Print and shaded views of the part. All mm, measured from the part's lowest x, y and z. Round coordinates to 2 decimals unless told otherwise and drop trailing zeros. Loops run counter-clockwise (first coordinate to the right, second up) from the corner with the lowest first, then second, coordinate; pieces in that order, holes last. Notation, with made-up numbers: (64.5, 35.25) -> (68.5, 35.25) arc R19 ccw to (68.5, 69.25) -> close; hole circle Ø4 at (17, 38.25). An arc over 180 degrees is marked (long way). Answer as CSV lines item,"result".
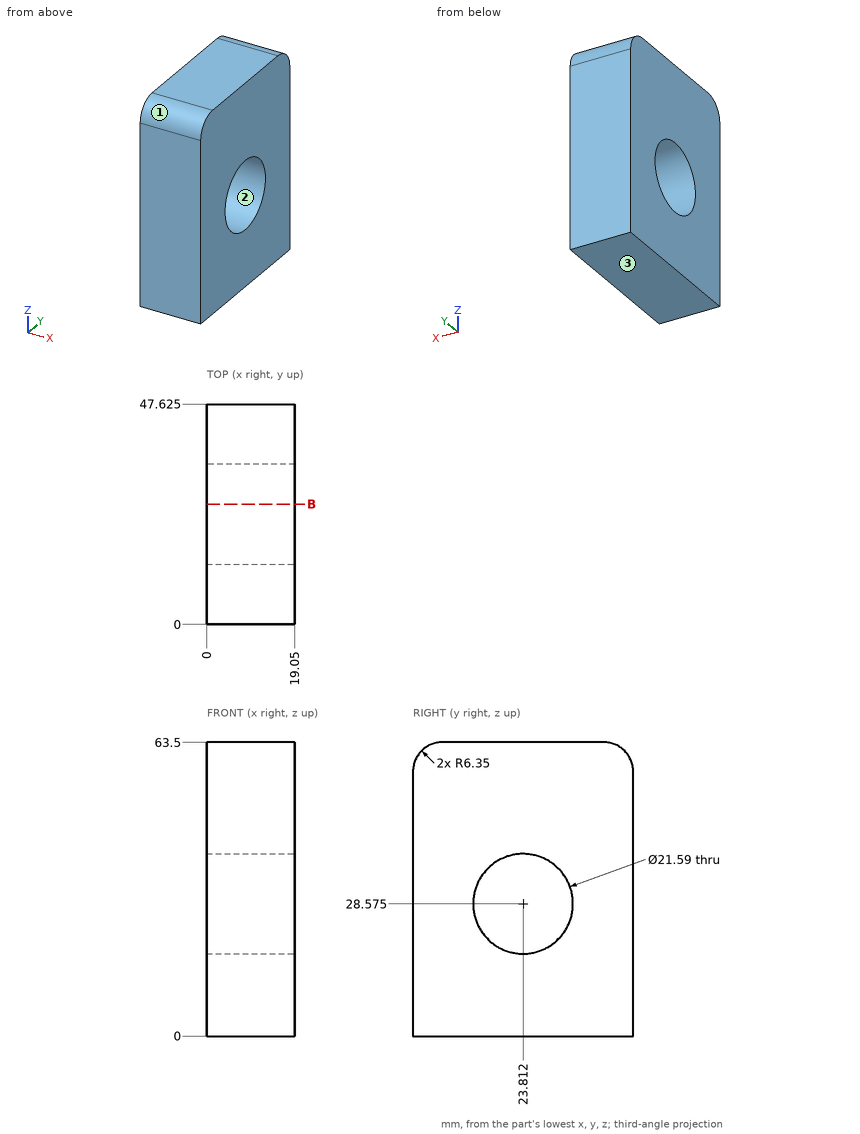
Q1. Drill centre lines: line 1 along Y through (x, z) = (7, 31.5) (1 decimal); line 2 along Z through (x, y) = (9, 22); line 3 along Y through (x, z) = (13, 36.5) (1 decimal). Where is each one in solid material? Low to high.
Geometry results:
line 1,"0 to 13.4, 34.2 to 47.6"
line 2,"0 to 17.93, 39.22 to 63.5"
line 3,"0 to 16.5, 31.1 to 47.6"
Q2. Drop a flat-ended pin along its axis: P1, Ø1, axis at y = 14, z = 26, coming from the +X side. Give the stop position or say it passes through.
Geometry results:
P1,"through"
Q3. Saw through at B-B, the plane y = 26. Write the cut outline in (x, z), then the cut area to 3 significant figures.
Geometry results:
outline,"(0, 0) -> (19.05, 0) -> (19.05, 18) -> (0, 18) -> close; (0, 39.15) -> (19.05, 39.15) -> (19.05, 63.5) -> (0, 63.5) -> close"
area,"807 mm2"
Q4. Two-plate mould, pull along Y, no slides. Class the marked faces 1, 2 and 3: pulls with the +Y half, pulls with the -Y half, needs draft (parallel to the pull), parting line crosses it, or undercut.
Geometry results:
face 1,"pulls with the -Y half"
face 2,"undercut"
face 3,"needs draft"
